Verification items for the finished model (mm, model axes). Face numbers are marked on the shaded views. Round coordinates to 2 decimals unless told otherwise and drop trailing zeros. Order: outer loops, then holes, each group sorted by start corner. A loop starts at its lowest first (then second) coordinate and runs counter-clockwise, first axis right, second up. Notation, with made-up numbers: M -2,64 L 32,64 A35 ccw 32,98 Z; hole C 34,19 d3. An arc over 180 degrees is marked long. Use CSV: the item, a comma, the result in double quotes. Start each with the question number.
Q1. Sectioned sample at B-B (x = 0). Enter the section's corners in (y, z).
Q2. Gauge pin test, flat ends, axial feed: pin 1 Ø6 at (y, z) = (19.5, 19) entering from -X; pin 2 Ø1 at (y, z) = (15.5, -22) entering from -X; pin 3 Ø10 at (x, y) = (31, 23) entering from +Z. Record the tip position at first contact, or that the pin passes through.
Q3. Scan lines: line 1 (Z direction, x = 0, y = 15.5); line 2 (Y direction, x = -33.5, z = 34). Record each from-to range of solid material in increasing order.
Q4. Sectioned sample at A-A (z = 0). Enter the section's corners in (x, y).
Q5. Sectioned sample at C-C (y = 22.5). Enter the section's corners in (x, z).
Q6. Mould release check, pull along Z, two halves, no side actions. Record for the marked faces 1, 2 and 3: +Z half, -Z half, draft (parallel to the pull), parting line (faces both ways), or undercut.
Autodesk Inventor part; units mm, degrees
ref_plane "YZ Plane" through (0, 0, 0) normal (1, 0, 0) x (0, 1, 0)
ref_plane "XZ Plane" through (0, 0, 0) normal (0, 1, 0) x (-1, 0, 0)
ref_plane "XY Plane" through (0, 0, 0) normal (0, 0, 1) x (1, 0, 0)
sketch "Sketch1" plane through (0, 0, 0) normal (0, 1, 0) x (-1, 0, 0)
  circle A0 centre (0, 0) radius 50
  dimension "d0" = 100
extrude "Extrusion1" add sketch "Sketch1" along normal blind 5
sketch "Sketch2" plane through (0, 5, 0) normal (0, 1, 0) x (1, 0, 0)
  circle A0 centre (0, 0) radius 29
  dimension "d3" = 58
extrude "Extrusion2" add sketch "Sketch2" along normal blind 22
thread "Thread1"
fillet "Fillet1" radius 2 1 edges at (50, 5, 0)
sketch "Sketch3" plane through (0, 27, 0) normal (0, 1, 0) x (1, 0, 0)
  circle A0 centre (0, 0) radius 27
  dimension "d9" = 54
extrude "Extrusion3" cut sketch "Sketch3" against normal blind 100
properties part number "palmPlatform"
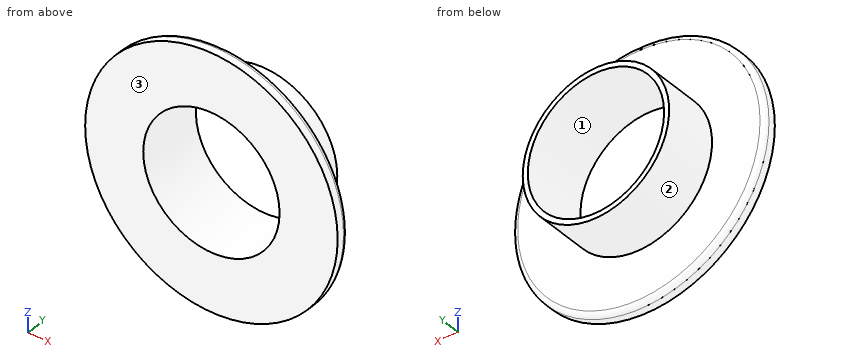
Verdict:
1,outline,"M 0,-50 L 3,-50 A2 ccw 5,-48 L 5,-29 L 27,-29 L 27,-27 L 0,-27 Z; M 0,27 L 27,27 L 27,29 L 5,29 L 5,48 A2 ccw 3,50 L 0,50 Z"
2,pin 1,"stops at x = -24.19"
2,pin 2,"stops at x = -19.46"
2,pin 3,"stops at z = 12.85"
3,line 1,"z = -29 to -27, 27 to 29"
3,line 2,"y = 0 to 5"
4,outline,"M -50,0 L -27,0 L -27,27 L -29,27 L -29,5 L -48,5 A2 ccw -50,3 Z; M 27,0 L 50,0 L 50,3 A2 ccw 48,5 L 29,5 L 29,27 L 27,27 Z"
5,outline,"C 0,0 d58; hole C 0,0 d54"
6,face 1,"undercut"
6,face 2,"parting line"
6,face 3,"draft"
